Print and shaded views of the part. All mm, measured from the part's lowest x, y and z. A direction names the side the tool comes from. Coordinates: 2 decimals unless noted, no trailing zeros. Order: outer loops, then holes, each group sorted by start corner. A loop starts at its lowest first (then second) coordinate and runs counter-clockwise, first axis right, second up. Notation, with made-up numbers: (61.25, 58.25) -> (66.25, 58.25) arc R36 cw to (66.25, 95.25) -> close; hole circle Ø3 at (32.25, -12). An arc over 180 degrees is marked (long way). Return JSON: item names as keys, results as strings. Group by question number.
1) Cut at C-C (y = 8). Write the cut outline in (x, z), and give its area (3 significant figures).
2) Flat gauge pin, fed straight in: pin 1 (2.5 mm diameter, centred on x = 4.5, z = 5.5, fed in from -Y). Where does the tip first touch, or does it go through?
3) Which spindle directions (+Z, -Z, +X, -X, +Y, -Y) get a long thin tool onto all of the face, cutting with end or side? Do the marked faces 4 and 5. Say none if no direction does.
4) Cut at D-D (x = 0.5). Write the cut outline in (y, z).
5) Cut at A-A (x = 5). Write the cut outline in (y, z).
6) Probe line 1 (Z direction, x = 8, y = 8.75); line 2 (Y direction, x = 5, z = 0.75); line 3 (Y direction, x = 2.75, z = 6). List the from-to ranges inside material, lowest first.
7) Cut at B-B (y = 5). Write the cut outline in (x, z).
8) Pull direction Z, two halves, no side cores. Call the marked faces 1, 2 and 3: +Z half, -Z half, draft (parallel to the pull), parting line (faces both ways), or undercut.
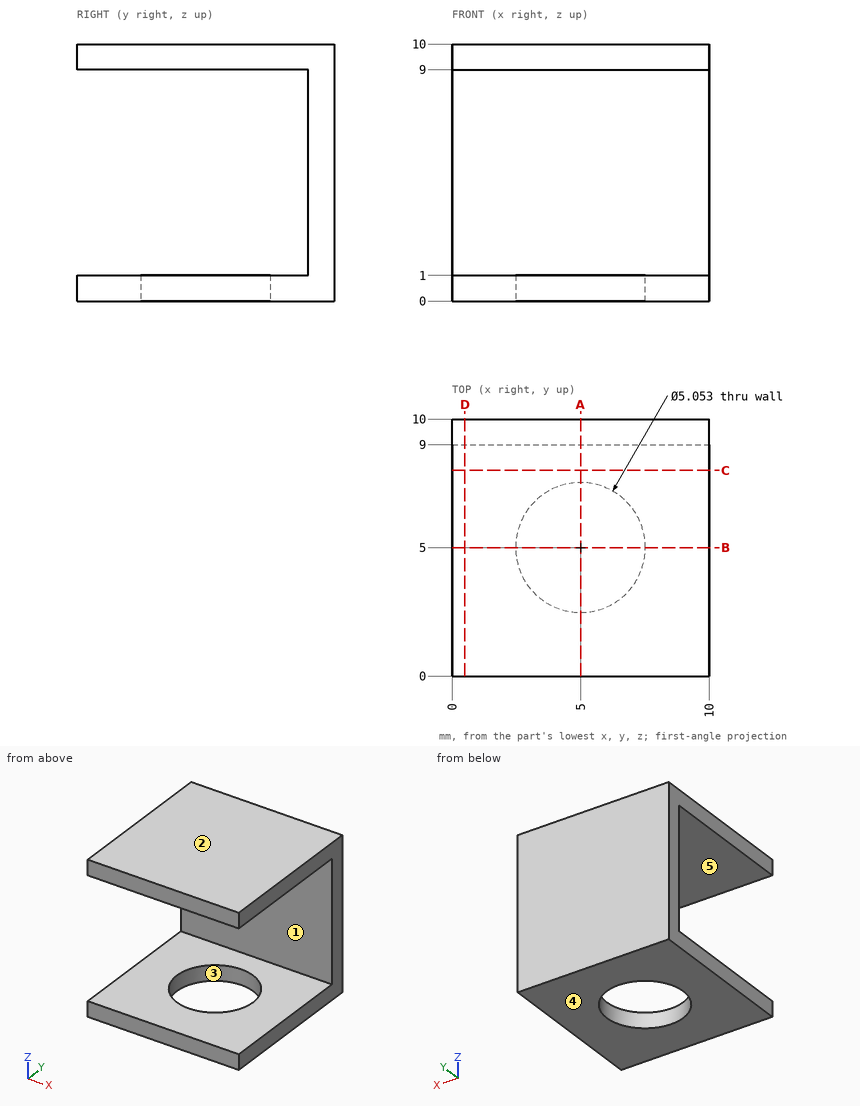
Answers below:
{
 "1": {"outline": "(0, 0) -> (10, 0) -> (10, 1) -> (0, 1) -> close; (0, 9) -> (10, 9) -> (10, 10) -> (0, 10) -> close", "area": "20.0 mm^2"},
 "2": {"pin 1": "stops at y = 9"},
 "3": {"face 4": "-Z, +X, -X, +Y, -Y", "face 5": "+X, -X, -Y"},
 "4": {"outline": "(0, 0) -> (10, 0) -> (10, 10) -> (0, 10) -> (0, 9) -> (9, 9) -> (9, 1) -> (0, 1) -> close"},
 "5": {"outline": "(0, 0) -> (2.47, 0) -> (2.47, 1) -> (0, 1) -> close; (0, 9) -> (9, 9) -> (9, 1) -> (7.53, 1) -> (7.53, 0) -> (10, 0) -> (10, 10) -> (0, 10) -> close"},
 "6": {"line 1": "z = 0 to 1, 9 to 10", "line 2": "y = 0 to 2.47, 7.53 to 10", "line 3": "y = 9 to 10"},
 "7": {"outline": "(0, 0) -> (2.47, 0) -> (2.47, 1) -> (0, 1) -> close; (0, 9) -> (10, 9) -> (10, 10) -> (0, 10) -> close; (7.53, 0) -> (10, 0) -> (10, 1) -> (7.53, 1) -> close"},
 "8": {"face 1": "undercut", "face 2": "+Z half", "face 3": "draft"}
}
